from build123d import *

# Parameters (mm, degrees)
SKETCH1_W           = 16.51
SKETCH1_H           = 17.4752
BOSS_EXTRUDE1_DEPTH = 1.27
SKETCH2_R           = 0.9525
CUT_EXTRUDE1_DEPTH  = 25.074376732
SKETCH4_W           = 1.27
SKETCH4_H           = 10.8204
CUT_EXTRUDE2_DEPTH  = 3.7592
SKETCH5_W           = 1.27
SKETCH5_H           = 4.064
CUT_EXTRUDE3_DEPTH  = 4.3688


with BuildPart() as part:
    # Sketch1 → Boss-Extrude1 (new body)
    with BuildSketch(Plane(origin=(0, 0, 0), x_dir=(0, 0, -1), z_dir=(1, 0, 0))):
        with Locations((-8.255, 8.7376)):
            Rectangle(SKETCH1_W, SKETCH1_H)
    extrude(amount=BOSS_EXTRUDE1_DEPTH)

    # Sketch2 → Cut-Extrude1 (cut, through all)
    with BuildSketch(Plane(origin=(1.27, 0, 0), x_dir=(0, 0, -1), z_dir=(1, 0, 0))):
        with Locations((-1.651, 14.9352)):
            Circle(SKETCH2_R)
    extrude(amount=-CUT_EXTRUDE1_DEPTH, mode=Mode.SUBTRACT)

    # Sketch4 → Cut-Extrude2 (cut)
    with BuildSketch(Plane(origin=(0, 0, 0), x_dir=(-1, 0, 0), z_dir=(0, 0, -1))):
        with Locations((-0.635, 5.4102)):
            Rectangle(SKETCH4_W, SKETCH4_H)
    extrude(amount=-CUT_EXTRUDE2_DEPTH, mode=Mode.SUBTRACT)

    # Sketch5 → Cut-Extrude3 (cut)
    with BuildSketch(Plane(origin=(0, 0, 3.7592), x_dir=(-1, 0, 0), z_dir=(0, 0, -1))):
        with Locations((-0.635, 8.7884)):
            Rectangle(SKETCH5_W, SKETCH5_H)
    extrude(amount=-CUT_EXTRUDE3_DEPTH, mode=Mode.SUBTRACT)


solid = part.part
Model file for the job. Use its own axes, mm. A direction names the side the tool comes from. Round coordinates to 2 decimals unless told otherwise and drop trailing zeros. Loops run counter-clockwise (first coordinate to the right, second up) from the corner with the lowest first, then second, coordinate; pieces in that order, holes last. Notation, with made-up numbers: M -1.5,34.5 L 19.5,34.5 A10 ccw 19.5,49.5 Z; hole C 61.25,23 d5. An arc over 180 degrees is marked long. One line per question, with ' | ' between items.
1) Drill centre lines: line 1 along Y through (x, z) = (0.4, 6.5); line 2 along Z through (x, y) = (0.45, 10.75); line 3 along Z through (x, y) = (0.8, 5.5). Where is each one in solid material? Low to high.
Solved:
line 1: y = 0 to 6.76, 10.82 to 17.48 | line 2: z = 8.13 to 16.51 | line 3: z = 3.76 to 16.51
2) Band-saw the part on D-D (y = 10). Give the cut face in (x, z).
Solved:
outline: M 0,8.13 L 1.27,8.13 L 1.27,16.51 L 0,16.51 Z
3) Flat gauge pins, fed straight in: pin 1 (0.6 mm diameter, centred on x = 1, y = 8.5, fed in from -Z); pin 2 (1.7 mm diameter, centred on y = 14.94, z = 1.65, fed in from +X). Where does each tip first touch, or does it go through?
Solved:
pin 1: stops at z = 8.13 | pin 2: passes through
4) Band-saw the part on A-A (z = 7). Give the cut face in (x, y), then the cut area to 3 significant figures.
Solved:
outline: M 0,0 L 1.27,0 L 1.27,6.76 L 0,6.76 Z; M 0,10.82 L 1.27,10.82 L 1.27,17.48 L 0,17.48 Z | area: 17.0 mm²
5) 3-axis set-ups, long thin cutter, end or side, ignore diameter. For faces 1 (the flat face through (1, 3, 3.759)), 2 (the flat face through (1, 9, 8.128)), 3 (the flat face through (0, 9, 10)): which of +Z, -Z, +X, -X, +Y, -Y reach the whole face in a straight line?
Solved:
face 1: -Z, +X, -X, -Y | face 2: -Z, +X, -X | face 3: +Z, -Z, -X, +Y, -Y
6) Band-saw the part on B-B (x = 0.5). Give the cut face in (y, z) (1 decimal).
Solved:
outline: M 0,3.8 L 6.8,3.8 L 6.8,8.1 L 10.8,8.1 L 10.8,0 L 17.5,0 L 17.5,16.5 L 0,16.5 Z; hole C 14.9,1.7 d1.9
7) Band-saw the part on C-C (y = 14.5). Give the cut face in (x, z).
Solved:
outline: M 0,0 L 1.27,0 L 1.27,0.8 L 0,0.8 Z; M 0,2.5 L 1.27,2.5 L 1.27,16.51 L 0,16.51 Z
8) Mould opens along Y. For faces 4 (the flat face through (1, 0, 10)), 5 (the flat face through (1, 10.82, 4)), 6 (the flat face through (1, 9, 16.51)) say: +Y half, -Y half, draft (parallel to the pull), parting line (faces both ways), or undercut.
Solved:
face 4: -Y half | face 5: undercut | face 6: draft
